Can you work these out from the model? Positions are in its coordinate system, mm. A direction names the side the tool comes from. Round coordinates to 2 decimals unless told otherwise and drop trailing zeros. Loops run counter-clockwise (first coordinate to the right, second up) from the corner with the lowest first, then second, coordinate; pieces in that order, holes last.
(1) I want a section at B-B on z = 17.75. Write out the boundary of the cut face in (x, y).
(2) Thinking about a two-plate mould opening in Z: for faces 4 (the face through (-30, -9.3, 14)), 5 (the face through (-24.3, -1.45, 1.6)), 6 (the face through (-31.89, -8.09, 10.4)), which applies, released by +Z, released by -Z, zero draft, split by the parting line, or undercut?
(3) If I drill on line 1 along Z through (x, y) = (16.5, -5); line 2 along X through (y, z) = (-3, 0.25); line 3 along X through (y, z) = (-12.5, 6), over which ranges is the centre line in solid material (lowest first)?
(4) Which directions (+Z, -Z, +X, -X, +Y, -Y) give clear straight access to the entire face, cutting with the end or side of a thin tool? Please do faces 1 (the face through (23, -13.5, 2)), 2 (the face through (23, 4.5, 2)), 3 (the face through (-29.205, -8.24, 13.291)).
(5) I want a section at C-C on x = 3.5. Write out the boundary of the cut face in (y, z), plus the area to 3 significant figures.
(6) I want a section at A-A on x = -25.5. Write out the boundary of the cut face in (y, z), plus the area to 3 significant figures.
(7) Will these pins go through, and if not, where does the flat tip stop? pin 1 Ø3 at (x, z) = (-30, 17.5) entering from +Y; pin 2 Ø6 at (x, y) = (5.5, 7) entering from +Z; pin 3 Ø4 at (y, z) = (-9, 3) entering from -X.
from build123d import *

# Parameters (mm, degrees)
CROQUIS1_W              = 43
CROQUIS1_H              = 35
BRIDA_BASE1_DEPTH       = 1.5
CROQUIS6_W              = 59.566817112
CROQUIS6_H              = 45.88022185
CORTAR_EXTRUIR1_DEPTH   = 10
BRIDA_DE_ARISTA1_DEPTH  = 18
BRIDA_DE_ARISTA2_DEPTH  = 12
CORTAR_EXTRUIR2_DEPTH   = 10
SALIENTE_EXTRUIR1_DEPTH = 1.5
CORTAR_EXTRUIR3_DEPTH   = 10
BRIDA_DE_ARISTA3_DEPTH  = 15.985281374


# Sheet-metal steps are written as plain solids
with BuildPart() as part:
    # Croquis1 → Brida base1 (new body)
    with BuildSketch(Plane.XY):
        Rectangle(CROQUIS1_W, CROQUIS1_H)
    extrude(amount=-BRIDA_BASE1_DEPTH)

    # Croquis6 → Cortar-Extruir1 (cut)
    with BuildSketch(Plane.XY):
        Rectangle(CROQUIS6_W, CROQUIS6_H)
        Polygon((19.5, -17.5), (21.5, -13.5), (21.5, 4.5), (13.260768396, 9.49227982), (0, 17.5), (-12.711890801, 9.791095082), (-19.5, -1.45), (-21.5, -1.45), (-21.5, -13.45), (-17.684098087, -13.45), (-11, -17.5), align=None, mode=Mode.SUBTRACT)
    extrude(amount=-CORTAR_EXTRUIR1_DEPTH, mode=Mode.SUBTRACT)

    # Brida de arista1 section (across the edge) → Brida de arista1 (add)
    with BuildSketch(Plane(origin=(22.2366, -13.5, 0), x_dir=(-1, 0, 0), z_dir=(0, 1, 0))):
        with BuildLine():
            Line((-1.5, 0.7366), (-1.5, 4.5))
            Line((-1.5, 4.5), (0, 4.5))
            Line((0, 4.5), (0, 0.7366))
            ThreePointArc((0, 0.7366), (0.215745145, 0.215745145), (0.7366, 0))
            Line((0.7366, 0), (0.7366, -1.5))
            ThreePointArc((0.7366, -1.5), (-0.844915027, -0.844915027), (-1.5, 0.7366))
        make_face()
    extrude(amount=BRIDA_DE_ARISTA1_DEPTH)

    # Brida de arista2 section (across the edge) → Brida de arista2 (add)
    with BuildSketch(Plane(origin=(-21.80510971, -1.45, 0), x_dir=(0.7071067811865438, 0, 0.7071067811865512), z_dir=(0, -1, 0))):
        with BuildLine():
            Line((-1.5, 0.30510971), (-1.5, 20.378679656))
            Line((-1.5, 20.378679656), (0, 20.378679656))
            Line((0, 20.378679656), (0, 0.30510971))
            ThreePointArc((0, 0.30510971), (0.056070336, 0.023225094), (0.215745145, -0.215745145))
            Line((0.215745145, -0.215745145), (-0.844915027, -1.276405317))
            ThreePointArc((-0.844915027, -1.276405317), (-1.329748962, -0.550800055), (-1.5, 0.30510971))
        make_face()
    extrude(amount=BRIDA_DE_ARISTA2_DEPTH)

    # Croquis13 → Cortar-Extruir2 (cut)
    with BuildSketch(Plane(origin=(-11.963215027, 0, -11.963215027), x_dir=(-0.7071067811865511, 0, 0.707106781186544), z_dir=(-0.707106781186544, 0, -0.7071067811865511))):
        Polygon((35.797220597, -1.45), (21.51312871, -15.734091887), (35.797220597, -15.734091887), align=None)
    extrude(amount=-CORTAR_EXTRUIR2_DEPTH, mode=Mode.SUBTRACT)

    # Croquis14 → Saliente-Extruir1 (add)
    with BuildSketch(Plane(origin=(-11.963215027, 0, -11.963215027), x_dir=(-0.7071067811865511, 0, 0.707106781186544), z_dir=(-0.707106781186544, 0, -0.7071067811865511))):
        Polygon((23.797220597, -1.45), (30.161181628, 4.913961031), (36.161181628, -1.086038969), (35.797220597, -1.45), align=None)
    extrude(amount=-SALIENTE_EXTRUIR1_DEPTH)

    # Croquis15 → Cortar-Extruir3 (cut)
    with BuildSketch(Plane(origin=(-11.963215027, 0, -11.963215027), x_dir=(-0.7071067811865511, 0, 0.707106781186544), z_dir=(-0.707106781186544, 0, -0.7071067811865511))):
        Polygon((30.161181628, 4.913961031), (36.161181628, -1.086038969), (35.100521456, -2.146699141), (29.100521456, 3.853300859), align=None)
    extrude(amount=-CORTAR_EXTRUIR3_DEPTH, mode=Mode.SUBTRACT)

    # Brida de arista3 section (across the edge) → Brida de arista3 (add)
    with BuildSketch(Plane(origin=(-36.0906716, -2.667553996, 14.28556189), x_dir=(0.5000000000000052, 0.7071067811865475, -0.499999999999995), z_dir=(0.5000000000000028, -0.7071067811865477, -0.49999999999999717))):
        with BuildLine():
            Line((-1.5, 0.7366), (-1.5, 7.5))
            Line((-1.5, 7.5), (0, 7.5))
            Line((0, 7.5), (0, 0.7366))
            ThreePointArc((0, 0.7366), (0.215745145, 0.215745145), (0.7366, 0))
            Line((0.7366, 0), (0.7366, -1.5))
            ThreePointArc((0.7366, -1.5), (-0.844915027, -0.844915027), (-1.5, 0.7366))
        make_face()
    extrude(amount=BRIDA_DE_ARISTA3_DEPTH)


solid = part.part
Filled sheet:
1. outline: (-34.13, -3.73) - (-28.95, -7.39) - (-28.95, -5.27) - (-32.63, -2.67) - close
2. face 4: released by +Z
2. face 5: zero draft
2. face 6: undercut
3. line 1: z = -1.5 to 0
3. line 2: x = -24.18 to -22.06, 22.05 to 23.68
3. line 3: x = -29.87 to -27.81
4. face 1: +Z, -Z, +X, -Y
4. face 2: +Z, -Z, +X, +Y
4. face 3: +X, +Y
5. outline: (-17.5, -1.5) - (15.39, -1.5) - (15.39, 0) - (-17.5, 0) - close
5. area: 49.3 mm2
6. outline: (-15.03, 10.39) - (-13.97, 8.89) - (-10.15, 14.3) - (-12.27, 14.3) - close; (-13.45, 1.57) - (-1.45, 1.57) - (-1.45, 3.69) - (-13.45, 3.69) - close
6. area: 35.3 mm2
7. pin 1: stops at y = -3.2
7. pin 2: stops at z = 0
7. pin 3: stops at x = -28.93
